Read the model definition and answer for the solid it produces. Units are mm, in the model's axes. A direction names the side the tool comes from. Coordinates: 2 decimals unless noted, no trailing zeros. Loops run counter-clockwise (first coordinate to the right, second up) from the corner with the lowest first, then second, coordinate; pieces in that order, holes last.
from build123d import *

# Parameters (mm, degrees)
SKETCH1_R           = 5.55625
BOSS_EXTRUDE1_DEPTH = 5.08
SKETCH2_R           = 3.175
BOSS_EXTRUDE2_DEPTH = 50.8
FILLET1_R           = 0.508


with BuildPart() as part:
    # Sketch1 → Boss-Extrude1 (new body)
    with BuildSketch(Plane.XY):
        Circle(SKETCH1_R)
        Polygon((2.794, 1.613116652), (0, 3.226233304), (-2.794, 1.613116652), (-2.794, -1.613116652), (0, -3.226233304), (2.794, -1.613116652), align=None, mode=Mode.SUBTRACT)
    extrude(amount=BOSS_EXTRUDE1_DEPTH)

    # Sketch2 → Boss-Extrude2 (add)
    with BuildSketch(Plane.XY.offset(5.08)):
        Circle(SKETCH2_R)
    extrude(amount=BOSS_EXTRUDE2_DEPTH)

    # Fillet1
    fillet1_edges = [part.edges().sort_by_distance(p)[0] for p in [
        (-3.175, 0, 55.88),
    ]]
    fillet(fillet1_edges, radius=FILLET1_R)


solid = part.part
Item 1: Find the intervals of material crossed by line 1 along Z through (x, y) = (-4, -2.25); line 2 along Z through (x, y) = (-1.5, -0.75); line 3 along Y through (x, z) = (-2.25, 4.5), in increasing order.
Numbers:
line 1: z = 0 to 5.08
line 2: z = 5.08 to 55.88
line 3: y = -5.08 to -1.93, 1.93 to 5.08
Item 2: A cutting plane is placed at D-D on y = 3.75. Determine the outline of the cut face in (x, z), then the cut area to 3 significant figures.
Numbers:
outline: (-4.1, 0) - (4.1, 0) - (4.1, 5.08) - (-4.1, 5.08) - close
area: 41.7 mm2
Item 3: A cutting plane is placed at C-C on x = -4.5. Determine the outline of the cut face in (y, z).
Numbers:
outline: (-3.26, 0) - (3.26, 0) - (3.26, 5.08) - (-3.26, 5.08) - close
Item 4: A cutting plane is placed at B-B on z = 25. Determine the outline of the cut face in (x, y) (3 decimals), then the cut area to 3 significant figures.
Numbers:
outline: circle Ø6.35 at (0, 0)
area: 31.7 mm2
Item 5: Given pin 1 (1.5 mm diameter, centred on x = -4, y = 2, fed in from +Z); pin 2 (5 mm diameter, centred on x = 3.5, y = 3.5, fed in from -Z); pin 3 (5 mm diameter, centred on y = 1, z = 18.5, fed in from +X) (3 decimals); pin 4 (6 mm diameter, centred on x = -4, z = 32, fed in from +Y), each flat-ended and moving along its own axis, determine where each tip first touches the part or whether it passes through.
Numbers:
pin 1: stops at z = 5.08
pin 2: stops at z = 0
pin 3: stops at x = 3.175
pin 4: stops at y = 3.01
Item 6: A cutting plane is placed at A-A on y = 0. Determine the outline of the cut face in (x, z) (3 decimals).
Numbers:
outline: (-5.556, 0) - (-2.794, 0) - (-2.794, 5.08) - (2.794, 5.08) - (2.794, 0) - (5.556, 0) - (5.556, 5.08) - (3.175, 5.08) - (3.175, 55.372) arc R0.508 ccw to (2.667, 55.88) - (-2.667, 55.88) arc R0.508 ccw to (-3.175, 55.372) - (-3.175, 5.08) - (-5.556, 5.08) - close
Item 7: Which of the six approach directions +Z, -Z, +X, -X, +Y, -Y give full straight-line access (tool end or side, diameter ignored) to faces 1 (the face through (-2.794, 0, 3)), 2 (the face through (0, 0, 55.88)), 3 (the face through (-0.69, -3.1, 29.87))?
Numbers:
face 1: -Z
face 2: +Z, +X, -X, +Y, -Y
face 3: +Z
